Here's the drawing with two shaded views (mm, measured from the low corner). I have some questions. A direction names the side the tool comes from. Give positions to 0.01 mm unless a question says otherwise; leave off trailing zeros. Write each loop counter-clockwise with the first axis right and the second up, starting at its lowest first coordinate (ties: lowest second). Pieces come first, ordered by that corner, then holes. Notation, with made-up numbers: (26.25, 46) -> (46.25, 46) arc R26 cw to (46.25, 68) -> close; hole circle Ø4 at (-24, 27.25). An arc over 180 degrees is marked (long way). One line per item, written item: value.
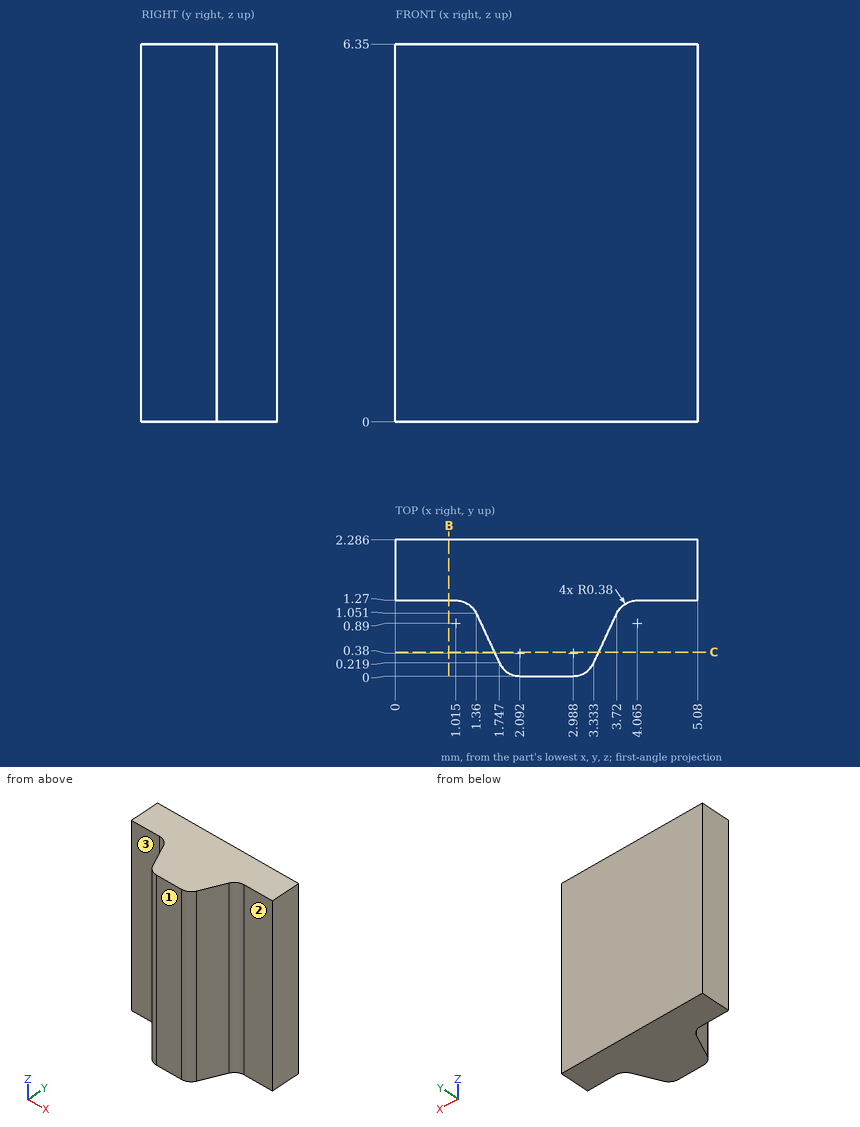
1) If we section it at B-B (x = 0.9): Write out the boundary of the cut face in (y, z).
Answer list:
outline: (1.27, 0) -> (2.29, 0) -> (2.29, 6.35) -> (1.27, 6.35) -> close
2) For the marked faces 1, 2 and 3, which set-ups out of +Z, -Z, +X, -X, +Y, -Y let a thin tool reach every point of the face, with its end or its side?
Answer list:
face 1: +Z, -Z, +X, -X, -Y
face 2: +Z, -Z, +X, -Y
face 3: +Z, -Z, -X, -Y
3) If we section it at C-C (y = 0.4): Write out the boundary of the cut face in (x, z).
Answer list:
outline: (1.66, 0) -> (3.42, 0) -> (3.42, 6.35) -> (1.66, 6.35) -> close
4) I need wall thicknesses on L1, parallel to Y at x = 0.4, z = 1.25; L2, parallel to Y at x = 1.75, z = 4.75 (1 decimal); L3, parallel to X at y = 0.7, z = 1. Which ranges of each line are inside material? Lowest first, please.
Answer list:
L1: y = 1.27 to 2.29
L2: y = 0.2 to 2.3
L3: x = 1.52 to 3.56
5) Will this pin go through, and if not, where does the flat tip stop? pin 1 (1.1 mm diameter, centred on x = 5, z = 4, fed in from -Y).
Answer list:
pin 1: stops at y = 1.27
